```python
from build123d import *

# Parameters (mm, degrees)
SKETCH_W        = 59
SKETCH_H        = 60
PAD_DEPTH       = 14
SKETCH001_R     = 7.6
POCKET_DEPTH    = 60.001
SKETCH002_R     = 1.75
POCKET001_DEPTH = 14.001
POCKET002_DEPTH = 11
SKETCH004_R     = 2.25
POCKET003_DEPTH = 14.001
SKETCH008_R     = 4.1
POCKET005_DEPTH = 20
SKETCH010_W     = 20
SKETCH010_H     = 25
POCKET006_DEPTH = 5
SKETCH011_R     = 2.25
POCKET007_DEPTH = 10
CHAMFER_SIZE    = 3
POCKET008_DEPTH = 4


with BuildPart() as part:
    # Sketch → Pad (new body)
    with BuildSketch(Plane.XY):
        with Locations((19.5, 0)):
            Rectangle(SKETCH_W, SKETCH_H)
    extrude(amount=PAD_DEPTH)

    # Sketch001 → Pocket (cut, through all)
    with BuildSketch(Plane.XZ.offset(30)):
        with Locations((0, 14)):
            Circle(SKETCH001_R)
    extrude(amount=-POCKET_DEPTH, mode=Mode.SUBTRACT)

    # Sketch002 → Pocket001 (cut, through all)
    with BuildSketch(Plane.XY.offset(14)):
        with Locations((-6, 27)):
            Circle(SKETCH002_R)
        with Locations((-6, -27)):
            Circle(SKETCH002_R)
        with Locations((6, 27)):
            Circle(SKETCH002_R)
        with Locations((6, -27)):
            Circle(SKETCH002_R)
        with Locations((6, 0)):
            Circle(SKETCH002_R)
        with Locations((-6, 0)):
            Circle(SKETCH002_R)
    extrude(amount=-POCKET001_DEPTH, mode=Mode.SUBTRACT)

    # Sketch003 → Pocket002 (cut)
    with BuildSketch(Plane.XY.offset(14)):
        with BuildLine():
            Line((10, 35), (10, -35))
            Line((10, -35), (32, -35))
            Line((32, -35), (32, -17.246794))
            ThreePointArc((32, -17.246794), (35.044647, -14.065445), (36.736695, -10))
            Line((36.736695, -10), (56.736695, -10))
            Line((56.736695, -10), (56.736695, 10))
            Line((56.736695, 10), (36.736695, 10))
            ThreePointArc((36.736695, 10), (35.044647, 14.065445), (32, 17.246794))
            Line((32, 17.246794), (32, 35))
            Line((32, 35), (10, 35))
        make_face()
    extrude(amount=-POCKET002_DEPTH, mode=Mode.SUBTRACT)

    # Sketch004 → Pocket003 (cut, through all)
    with BuildSketch(Plane(origin=(0, 0, 0), x_dir=(1, 0, 0), z_dir=(0, 0, -1))):
        with Locations((25, 7.5)):
            Circle(SKETCH004_R)
        with Locations((25, -7.5)):
            Circle(SKETCH004_R)
    extrude(amount=-POCKET003_DEPTH, mode=Mode.SUBTRACT)

    # Sketch008 → Pocket005 (cut)
    with BuildSketch(Plane.YZ.offset(49)):
        with Locations((-20, 14)):
            Circle(SKETCH008_R)
        with Locations((20, 14)):
            Circle(SKETCH008_R)
    extrude(amount=-POCKET005_DEPTH, mode=Mode.SUBTRACT)

    # Sketch010 → Pocket006 (cut)
    with BuildSketch(Plane.YZ.offset(49)):
        with Locations((0, 6.5)):
            Rectangle(SKETCH010_W, SKETCH010_H)
    extrude(amount=-POCKET006_DEPTH, mode=Mode.SUBTRACT)

    # Sketch011 → Pocket007 (cut)
    with BuildSketch(Plane.XY.offset(14)):
        with Locations((40, 27)):
            Circle(SKETCH011_R)
        with Locations((40, 13)):
            Circle(SKETCH011_R)
        with Locations((40, -13)):
            Circle(SKETCH011_R)
        with Locations((40, -27)):
            Circle(SKETCH011_R)
    extrude(amount=-POCKET007_DEPTH, mode=Mode.SUBTRACT)

    # Chamfer
    chamfer_edges = [part.edges().sort_by_distance(p)[0] for p in [
        (49, -10, 8.5),
        (49, 10, 8.5),
    ]]
    chamfer(chamfer_edges, length=CHAMFER_SIZE)

    # Sketch012 → Pocket008 (cut)
    with BuildSketch(Plane(origin=(0, 0, 0), x_dir=(1, 0, 0), z_dir=(0, 0, -1))):
        Polygon((-4.412285, 29.750003), (-7.587715, 29.750003), (-9.17543, 27), (-7.587715, 24.249997), (-4.412285, 24.249997), (-2.82457, 27), align=None)
        Polygon((7.587715, 29.750003), (4.412285, 29.750003), (2.82457, 27), (4.412285, 24.249997), (7.587715, 24.249997), (9.17543, 27), align=None)
        Polygon((-4.412285, 2.750003), (-7.587715, 2.750003), (-9.17543, 0), (-7.587715, -2.750003), (-4.412285, -2.750003), (-2.82457, 0), align=None)
        Polygon((7.587715, 2.750003), (4.412285, 2.750003), (2.82457, 0), (4.412285, -2.750003), (7.587715, -2.750003), (9.17543, 0), align=None)
        Polygon((-4.412285, -24.249997), (-7.587715, -24.249997), (-9.17543, -27), (-7.587715, -29.750003), (-4.412285, -29.750003), (-2.82457, -27), align=None)
        Polygon((7.587715, -24.249997), (4.412285, -24.249997), (2.82457, -27), (4.412285, -29.750003), (7.587715, -29.750003), (9.17543, -27), align=None)
    extrude(amount=-POCKET008_DEPTH, mode=Mode.SUBTRACT)


solid = part.part
```
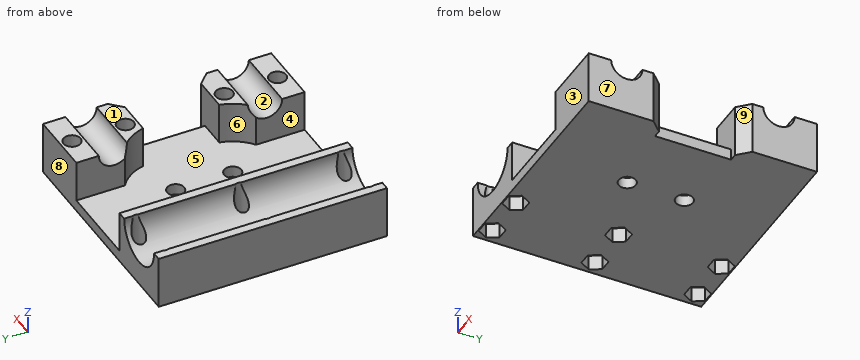
Could you check a few things on this model? Use its own coordinates, in mm. Face numbers are marked on the shaded views. A direction names the side the tool comes from. Give positions to 0.01 mm unless a question says otherwise; leave off trailing zeros. Loops run counter-clockwise (first coordinate to the right, second up) from the corner with the lowest first, then second, coordinate; pieces in that order, holes last. Notation, with made-up numbers: (34, 64) - (75, 64) arc R17 ccw to (75, 72) - close; hole circle Ø8 at (-4, -10.75). An arc over 180 degrees is marked (long way). Answer in a Markdown table with one row per item. Add a question column.
Q1. If we section it at D-D (x = 28.5): List the corners of the cut face in (y, z) for me, plus the area to 3 significant figures.
Q2. Which directions (+Z, -Z, +X, -X, +Y, -Y) give clear straight access to the entire face, cutting with the end or side of a thin tool? Please do the marked faces 1, 2, 3, 4 and 5.
Q3. If we section it at C-C (y = 20): List the corners of the cut face in (x, z) for me.
Q4. For pin 1 (7 mm diameter, centred on x = 40, y = -27, fed in from -Z); pin 2 (1.7 mm diameter, centred on x = -7.5, y = -1, fed in from -Z); pin 3 (4 mm diameter, centred on y = -4.5, z = 9.5, fed in from +X), each with a flat end and sliding along its axis, tell me the tip position at first contact or that it passes through.
Q5. If we section it at B-B (x = 40): List the corners of the cut face in (y, z) for me.
Q6. We'd pull the mould along Y, two halves only. Please class the marked faces 6, 7, 8 and 9: +Y half, -Y half, draft (parallel to the pull), parting line (faces both ways), or undercut.
Q7. If we section it at A-A (y = 7.5): List the corners of the cut face in (x, z) for me.
Q8. Please list where these lines run through material, in increasing order: L1, parallel to Y at x = 40, z = 7; L2, parallel to Y at x = -6, z = 7.25; L3, parallel to X at y = 21, z = 9.25. Write a range as from..to.
The answers:
| question | item | result |
|---|---|---|
| 1 | outline | (-30, 0) - (30, 0) - (30, 3) - (-30, 3) - close |
| 1 | area | 180 mm^2 |
| 2 | face 1 | +Z, +X, -X, +Y, -Y |
| 2 | face 2 | +Z, +X |
| 2 | face 3 | +Z, -Z, +X, -X, -Y |
| 2 | face 4 | +Z, +Y, -Y |
| 2 | face 5 | +Z |
| 3 | outline | (-10, 0) - (49, 0) - (49, 9.9) - (32, 9.9) - (32, 3) - (10, 3) - (10, 14) - (7.6, 14) arc R7.6 cw to (-7.6, 14) - (-10, 14) - close |
| 4 | pin 1 | stops at z = 0 |
| 4 | pin 2 | stops at z = 4 |
| 4 | pin 3 | stops at x = 10 |
| 5 | outline | (-30, 0) - (30, 0) - (30, 14) - (29.25, 14) - (29.25, 4) - (24.75, 4) - (24.75, 14) - (24.1, 14) arc R4.1 cw to (15.9, 14) - (15.25, 14) - (15.25, 4) - (10.75, 4) - (10.75, 14) - (10, 14) - (10, 3) - (-10, 3) - (-10, 14) - (-10.75, 14) - (-10.75, 4) - (-15.25, 4) - (-15.25, 14) - (-15.9, 14) arc R4.1 cw to (-24.1, 14) - (-24.75, 14) - (-24.75, 4) - (-29.25, 4) - (-29.25, 14) - (-30, 14) - close |
| 6 | face 6 | undercut |
| 6 | face 7 | draft |
| 6 | face 8 | +Y half |
| 6 | face 9 | undercut |
| 7 | outline | (-10, 0) - (22.75, 0) - (22.75, 3) - (10, 3) - (10, 14) - (7.6, 14) arc R7.6 cw to (-7.6, 14) - (-10, 14) - close; (27.25, 0) - (44, 0) - (44, 3) - (27.25, 3) - close |
| 8 | L1 | y = -30..-29.25, -24.75..-15.25, -10.75..-10, 10..10.75, 15.25..24.75, 29.25..30 |
| 8 | L2 | y = -30..-28.75, -25.25..-1.75, 1.75..25.25, 28.75..30 |
| 8 | L3 | x = -10..-5.93, 5.93..10, 32..49 |
